```python
from build123d import *

# Parameters (mm, degrees)
SKETCH1_R      = 2.54
EXTRUDE1_DEPTH = 20.574
SKETCH2_R      = 19.05
EXTRUDE2_DEPTH = 1.524
SKETCH3_R      = 3.175
EXTRUDE3_DEPTH = 20.574
EXTRUDE4_START = -36.068
EXTRUDE4_DEPTH = 36.068
FILLET1_R      = 2.54
EXTRUDE5_START = 14.986
SKETCH5_R      = 3.175
EXTRUDE5_DEPTH = 14.986
SKETCH6_R      = 1.07823
EXTRUDE6_DEPTH = 3.81


with BuildPart() as part:
    # Sketch1 → Extrude1 (new, symmetric)
    with BuildSketch(Plane.XY):
        with BuildLine():
            Line((-23.5712, 28.575), (23.5712, 28.575))
            ThreePointArc((23.5712, 28.575), (27.109420912, 27.109420912), (28.575, 23.5712))
            Line((28.575, 23.5712), (28.575, -23.5712))
            ThreePointArc((28.575, -23.5712), (27.109420912, -27.109420912), (23.5712, -28.575))
            Line((23.5712, -28.575), (-23.5712, -28.575))
            ThreePointArc((-23.5712, -28.575), (-27.109420912, -27.109420912), (-28.575, -23.5712))
            Line((-28.575, -23.5712), (-28.575, 23.5712))
            ThreePointArc((-28.575, 23.5712), (-27.109420912, 27.109420912), (-23.5712, 28.575))
        make_face()
        with Locations((-23.5712, 23.5712)):
            Circle(SKETCH1_R, mode=Mode.SUBTRACT)
        with Locations((23.5712, 23.5712)):
            Circle(SKETCH1_R, mode=Mode.SUBTRACT)
        with Locations((23.5712, -23.5712)):
            Circle(SKETCH1_R, mode=Mode.SUBTRACT)
        with Locations((-23.5712, -23.5712)):
            Circle(SKETCH1_R, mode=Mode.SUBTRACT)
    extrude(amount=EXTRUDE1_DEPTH, both=True)

    # Sketch2 → Extrude2 (add)
    with BuildSketch(Plane.XY.offset(20.574)):
        with Locations(Location((0, 0, 0), (0, 0, 180))):
            Circle(SKETCH2_R)
    extrude(amount=EXTRUDE2_DEPTH)

    # Sketch3 → Extrude3 (add)
    with BuildSketch(Plane.XY.offset(20.574)):
        Circle(SKETCH3_R)
    extrude(amount=EXTRUDE3_DEPTH)

    # Sketch4 → Extrude4 (cut)
    with BuildSketch(Plane(origin=(0, 0, -20.574), x_dir=(-1, 0, 0), z_dir=(0, 0, -1)).offset(EXTRUDE4_START)):
        with BuildLine():
            Line((-23.5712, 18.5674), (-28.575, 18.5674))
            Line((-28.575, 18.5674), (-28.575, 23.5712))
            ThreePointArc((-28.575, 23.5712), (-27.109420912, 27.109420912), (-23.5712, 28.575))
            Line((-23.5712, 28.575), (-18.5674, 28.575))
            Line((-18.5674, 28.575), (-18.5674, 23.5712))
            ThreePointArc((-18.5674, 23.5712), (-20.032979088, 20.032979088), (-23.5712, 18.5674))
        make_face()
        with BuildLine():
            Line((23.5712, 18.5674), (28.575, 18.5674))
            Line((28.575, 18.5674), (28.575, 23.5712))
            ThreePointArc((28.575, 23.5712), (27.109420912, 27.109420912), (23.5712, 28.575))
            Line((23.5712, 28.575), (18.5674, 28.575))
            Line((18.5674, 28.575), (18.5674, 23.5712))
            ThreePointArc((18.5674, 23.5712), (20.032979088, 20.032979088), (23.5712, 18.5674))
        make_face()
        with BuildLine():
            Line((23.5712, -18.5674), (28.575, -18.5674))
            Line((28.575, -18.5674), (28.575, -23.5712))
            ThreePointArc((28.575, -23.5712), (27.109420912, -27.109420912), (23.5712, -28.575))
            Line((23.5712, -28.575), (18.5674, -28.575))
            Line((18.5674, -28.575), (18.5674, -23.5712))
            ThreePointArc((18.5674, -23.5712), (20.032979088, -20.032979088), (23.5712, -18.5674))
        make_face()
        with BuildLine():
            Line((-18.5674, -23.5712), (-18.5674, -28.575))
            Line((-18.5674, -28.575), (-23.5712, -28.575))
            ThreePointArc((-23.5712, -28.575), (-27.109420912, -27.109420912), (-28.575, -23.5712))
            Line((-28.575, -23.5712), (-28.575, -18.5674))
            Line((-28.575, -18.5674), (-23.5712, -18.5674))
            ThreePointArc((-23.5712, -18.5674), (-20.032979088, -20.032979088), (-18.5674, -23.5712))
        make_face()
    extrude(amount=EXTRUDE4_DEPTH, mode=Mode.SUBTRACT)

    # Fillet1
    fillet1_edges = [part.edges().sort_by_distance(p)[0] for p in [
        (28.575, -18.5674, -2.54),
        (18.5674, -28.575, -2.54),
        (18.5674, 28.575, -2.54),
        (28.575, 18.5674, -2.54),
        (-28.575, 18.5674, -2.54),
        (-18.5674, 28.575, -2.54),
        (-18.5674, -28.575, -2.54),
        (-28.575, -18.5674, -2.54),
    ]]
    fillet(fillet1_edges, radius=FILLET1_R)

    # Sketch5 → Extrude5 (add)
    with BuildSketch(Plane(origin=(0, 0, -20.574), x_dir=(-1, 0, 0), z_dir=(0, 0, -1)).offset(EXTRUDE5_START)):
        with Locations(Location((0, 0, 0), (0, 0, 180))):
            Circle(SKETCH5_R)
    extrude(amount=-EXTRUDE5_DEPTH)

    # Sketch6 → Extrude6 (cut)
    with BuildSketch(Plane(origin=(0, 0, -20.574), x_dir=(-1, 0, 0), z_dir=(0, 0, -1))):
        with Locations((-23.0124, 0)):
            Circle(SKETCH6_R)
        with Locations((23.0124, 0)):
            Circle(SKETCH6_R)
    extrude(amount=-EXTRUDE6_DEPTH, mode=Mode.SUBTRACT)


solid = part.part
```
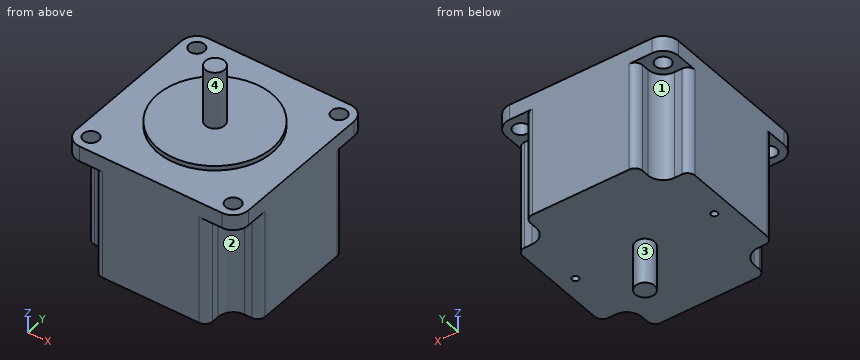
Here's how the part is built. I have some questions about the finished solid (model axes, mm). Face numbers are marked on the shaded views. A direction names the side the tool comes from. Coordinates: 2 decimals unless noted, no trailing zeros. Loops run counter-clockwise (first coordinate to the right, second up) from the corner with the lowest first, then second, coordinate; pieces in that order, holes last. Notation, with made-up numbers: (50, 70) -> (63, 70) arc R19 ccw to (63, 100) -> close; hole circle Ø2 at (87, -24). An arc over 180 degrees is marked (long way). Return JSON: item names as keys, results as strings.
1) If we section it at A-A, the plane x = 0: Write out the boundary of the cut face in (y, z) (3 decimals), then the cut area to 3 significant figures.
Results below:
{"outline": "(-28.575, -20.574) -> (-3.175, -20.574) -> (-3.175, -35.56) -> (3.175, -35.56) -> (3.175, -20.574) -> (28.575, -20.574) -> (28.575, 20.574) -> (19.05, 20.574) -> (19.05, 22.098) -> (3.175, 22.098) -> (3.175, 41.148) -> (-3.175, 41.148) -> (-3.175, 22.098) -> (-19.05, 22.098) -> (-19.05, 20.574) -> (-28.575, 20.574) -> close", "area": "2,630 mm²"}
2) If we section it at C-C, the plane y = 0: Write out the boundary of the cut face in (x, z) (3 decimals), then the cut area to 3 significant figures.
Results below:
{"outline": "(-28.575, -20.574) -> (-24.091, -20.574) -> (-24.091, -16.764) -> (-21.934, -16.764) -> (-21.934, -20.574) -> (-3.175, -20.574) -> (-3.175, -35.56) -> (3.175, -35.56) -> (3.175, -20.574) -> (21.934, -20.574) -> (21.934, -16.764) -> (24.091, -16.764) -> (24.091, -20.574) -> (28.575, -20.574) -> (28.575, 20.574) -> (19.05, 20.574) -> (19.05, 22.098) -> (3.175, 22.098) -> (3.175, 41.148) -> (-3.175, 41.148) -> (-3.175, 22.098) -> (-19.05, 22.098) -> (-19.05, 20.574) -> (-28.575, 20.574) -> close", "area": "2,610 mm²"}
3) If we section it at D-D, the plane x = 20: Write out the boundary of the cut face in (y, z) (3 decimals), then the cut area to 3 significant figures.
Results below:
{"outline": "(-28.575, 15.494) -> (-20.066, 15.494) -> (-20.066, -20.574) -> (20.066, -20.574) -> (20.066, 15.494) -> (28.575, 15.494) -> (28.575, 20.574) -> (-28.575, 20.574) -> close", "area": "1,740 mm²"}
4) Will these pins go through, and if not, where does the flat tip stop? pin 1 (1 mm diameter, centred on x = -14.5, y = 17.5, fed in from +Z); pin 2 (0.7 mm diameter, centred on y = 24.5, z = 5, fed in from -X); pin 3 (6.5 mm diameter, centred on x = -24, y = 20.5, fed in from -Z).
Results below:
{"pin 1": "z = 20.57", "pin 2": "x = -18.57", "pin 3": "z = -20.57"}
5) For the marked faces 1, 2, 3 and 4, which set-ups out of +Z, -Z, +X, -X, +Y, -Y let a thin tool reach every point of the face, with its end or its side?
Results below:
{"face 1": "-Z, -X, +Y", "face 2": "-Z, +X, -Y", "face 3": "-Z", "face 4": "+Z"}
6) If we section it at B-B, the plane z = 2: Write out the boundary of the cut face in (x, y) (3 decimals).
Results below:
{"outline": "(-28.575, -16.027) arc R2.54 ccw to (-26.035, -18.567) -> (-23.571, -18.567) arc R5.004 cw to (-18.567, -23.571) -> (-18.567, -26.035) arc R2.54 ccw to (-16.027, -28.575) -> (16.027, -28.575) arc R2.54 ccw to (18.567, -26.035) -> (18.567, -23.571) arc R5.004 cw to (23.571, -18.567) -> (26.035, -18.567) arc R2.54 ccw to (28.575, -16.027) -> (28.575, 16.027) arc R2.54 ccw to (26.035, 18.567) -> (23.571, 18.567) arc R5.004 cw to (18.567, 23.571) -> (18.567, 26.035) arc R2.54 ccw to (16.027, 28.575) -> (-16.027, 28.575) arc R2.54 ccw to (-18.567, 26.035) -> (-18.567, 23.571) arc R5.004 cw to (-23.571, 18.567) -> (-26.035, 18.567) arc R2.54 ccw to (-28.575, 16.027) -> close"}
7) I need wall thicknesses on line 1 (Z direction, x = -16.5, y = -0.5); line 2 (Z direction, x = -23, y = 11); line 3 (Y direction, x = -22.5, z = 12). Which ranges of each line are inside material? Lowest first, please. Write a range as from..to.
Results below:
{"line 1": "-20.57..22.1", "line 2": "-20.57..20.57", "line 3": "-18.68..18.68"}
